Source: CAD feature listing. Evaluate the final solid. Frame: model axes, mm. Face numbers are marked on the shaded views. A direction names the side the tool comes from. Round coordinates to 2 decimals unless told otherwise and drop trailing zeros. Order: outer loops, then holes, each group sorted by start corner. A loop starts at its lowest first (then second) coordinate and runs counter-clockwise, first axis right, second up. Notation, with made-up numbers: (26, -22.5) -> (44, -22.5) arc R32 ccw to (44, 14.5) -> close; hole circle Ø11 at (76.25, -21.75). An arc over 180 degrees is marked (long way). Write item = value, one per line. Start each with the question number.
(1) Ray query, line 1 (Y direction, x = -3, z = 6.25); line 2 (Y direction, x = -2, z = 11); line 3 (Z direction, x = 1, y = 21). Return the intervals inside material, ascending.
(2) Cut plane C-C on y = 1.5. Return the cut outline in (x, z).
(3) Cut plane D-D on y = 19.5. Return the cut outline in (x, z).
(4) Reachability of the marked faces 1, 2 and 3 from +Z, -Z, +X, -X, +Y, -Y: full face, straight path, thin tool, end or side. Return the list, or none.
(5) Cut plane A-A on x = 0. Return the cut outline in (y, z).
(6) Contact query for flat-ended pins moving along their axis: pin 1 Ø4 at (x, z) = (-5.5, -5.5) entering from +Y; pin 2 Ø8 at (y, z) = (17, -2) entering from +X; pin 3 Ø0.9 at (y, z) = (8.5, 8) entering from -X. Output: stop coordinate, or through.
(7) Cut plane B-B on z = 0.75. Return the cut outline in (x, y).
from build123d import *

# Parameters (mm, degrees)
SKETCH1_R           = 8.5
BOSS_EXTRUDE1_DEPTH = 9.5
SKETCH2_R           = 3
BOSS_EXTRUDE2_DEPTH = 15
SKETCH3_W           = 16.912520663
SKETCH3_H           = 13
BOSS_EXTRUDE3_DEPTH = 3
CUT_EXTRUDE2_DEPTH  = 24.774986856


with BuildPart() as part:
    # Sketch1 → Boss-Extrude1 (new body)
    with BuildSketch(Plane(origin=(0, 0, 0), x_dir=(1, 0, 0), z_dir=(0, 1, 0))):
        with Locations(Location((0, 0, 0), (0, 0, 270))):
            Circle(SKETCH1_R)
    extrude(amount=BOSS_EXTRUDE1_DEPTH)

    # Sketch2 → Boss-Extrude2 (add)
    with BuildSketch(Plane(origin=(0, 9.5, 0), x_dir=(1, 0, 0), z_dir=(0, 1, 0))):
        with Locations(Location((0, 0, 0), (0, 0, 270))):
            Circle(SKETCH2_R)
    extrude(amount=BOSS_EXTRUDE2_DEPTH)

    # Sketch3 → Boss-Extrude3 (add)
    with BuildSketch(Plane(origin=(0, 9.5, 0), x_dir=(1, 0, 0), z_dir=(0, 1, 0))):
        with Locations((0.043739668, -6.5)):
            Rectangle(SKETCH3_W, SKETCH3_H)
    extrude(amount=-BOSS_EXTRUDE3_DEPTH)

    # Sketch4 → Cut-Extrude2 (cut, through all)
    with BuildSketch(Plane.XZ.offset(-6.5)):
        with BuildLine():
            Line((-7.016472339, 13), (-7.016472339, 4.797824081))
            ThreePointArc((-7.016472339, 4.797824081), (-7.919608809, 3.087036818), (-8.412520663, 1.216345382))
            Line((-8.412520663, 1.216345382), (-8.412520663, 13))
            Line((-8.412520663, 13), (-7.016472339, 13))
        make_face()
        with BuildLine():
            Line((7.016472339, 13), (7.016472339, 4.797824081))
            ThreePointArc((7.016472339, 4.797824081), (8.120653141, 2.510974424), (8.5, 0))
            Line((8.5, 0), (8.5, 13))
            Line((8.5, 13), (7.016472339, 13))
        make_face()
    extrude(amount=-CUT_EXTRUDE2_DEPTH, mode=Mode.SUBTRACT)


solid = part.part
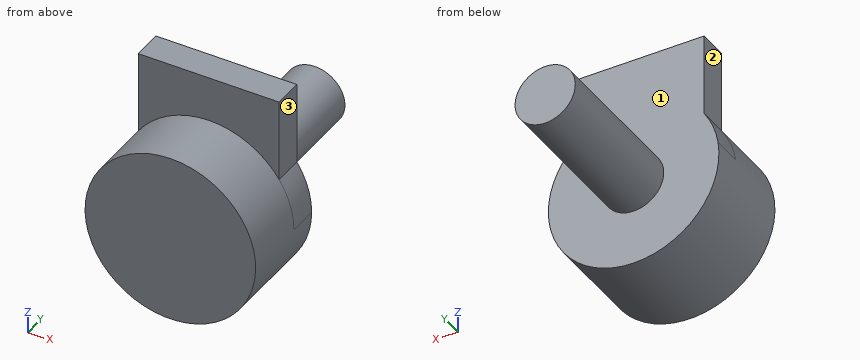
Evaluation:
q1.line_1 = 0 to 9.5
q1.line_2 = 6.5 to 9.5
q1.line_3 = -2.83 to 2.83
q2.outline = circle Ø17 at (0, 0)
q3.outline = circle Ø6 at (0, 0)
q4.face_1 = +Y
q4.face_2 = +Z, -X, +Y, -Y
q4.face_3 = +Z, +X, +Y, -Y
q5.outline = (0, -8.5) -> (9.5, -8.5) -> (9.5, -3) -> (24.5, -3) -> (24.5, 3) -> (9.5, 3) -> (9.5, 13) -> (6.5, 13) -> (6.5, 8.5) -> (0, 8.5) -> close
q6.pin_1 = 9.5
q6.pin_2 = 3
q6.pin_3 = -7.02
q7.outline = (-8.47, 0) -> (8.47, 0) -> (8.47, 9.5) -> (2.9, 9.5) -> (2.9, 24.5) -> (-2.9, 24.5) -> (-2.9, 9.5) -> (-8.47, 9.5) -> close
